Input: part model. Units: mm. Frame: model coordinates. A direction names the side the tool comes from. Give positions to 0.01 mm unless a question says otherwise; leave off trailing zeros. Loops run counter-clockwise (first coordinate to the right, second up) from the corner with the lowest first, then second, coordinate; pieces in that order, holes last.
from build123d import *
from OCP.BRepFilletAPI import BRepFilletAPI_MakeChamfer

# Parameters (mm, degrees)
SKETCH_1_W      = 60
SKETCH_1_H      = 30
EXTRUDE_1_DEPTH = 30
SKETCH_2_W      = 30
SKETCH_2_H      = 30
EXTRUDE_2_DEPTH = 80
EXTRUDE_3_DEPTH = 47
CHAMFER_1_SIZE  = 40
CHAMFER_1_SIZE2 = 7.053079228


with BuildPart() as part:
    # ｽｹｯﾁ1 → ﾎﾞｽ - 押し出し1 (new body)
    with BuildSketch(Plane(origin=(0, 0, 0), x_dir=(1, 0, 0), z_dir=(0, 1, 0))):
        with Locations((30, -15)):
            Rectangle(SKETCH_1_W, SKETCH_1_H)
    extrude(amount=EXTRUDE_1_DEPTH)

    # ｽｹｯﾁ2 → ﾎﾞｽ - 押し出し2 (add)
    with BuildSketch(Plane(origin=(0, 30, 0), x_dir=(1, 0, 0), z_dir=(0, 1, 0))):
        with Locations((15, -15)):
            Rectangle(SKETCH_2_W, SKETCH_2_H)
    extrude(amount=EXTRUDE_2_DEPTH)

    # ｽｹｯﾁ3 → ﾎﾞｽ - 押し出し3 (add)
    with BuildSketch(Plane(origin=(0, 110, 0), x_dir=(1, 0, 0), z_dir=(0, 1, 0))):
        Polygon((4.393398282, -15), (15, -4.393398282), (25.606601718, -15), (15, -25.606601718), align=None)
    extrude(amount=EXTRUDE_3_DEPTH)

    # 面取り1: one chamfer whose edges measure the first distance from different faces: ONE call of the kernel's chamfer builder (chamfer() names one face for all edges)
    chamfer_1_edges_1 = [part.edges().sort_by_distance(p)[0] for p in [
        (9.696699141, 157, 20.303300859),
    ]]
    chamfer_1_side_1 = [part.faces().sort_by_distance(p)[0] for p in [
        (9.696699141, 133.5, 20.303300859),
    ]]
    chamfer_1_edges_2 = [part.edges().sort_by_distance(p)[0] for p in [
        (20.303300859, 157, 20.303300859),
    ]]
    chamfer_1_side_2 = [part.faces().sort_by_distance(p)[0] for p in [
        (20.303300859, 133.5, 20.303300859),
    ]]
    chamfer_1_edges_3 = [part.edges().sort_by_distance(p)[0] for p in [
        (20.303300859, 157, 9.696699141),
    ]]
    chamfer_1_side_3 = [part.faces().sort_by_distance(p)[0] for p in [
        (20.303300859, 133.5, 9.696699141),
    ]]
    chamfer_1_edges_4 = [part.edges().sort_by_distance(p)[0] for p in [
        (9.696699141, 157, 9.696699141),
    ]]
    chamfer_1_side_4 = [part.faces().sort_by_distance(p)[0] for p in [
        (9.696699141, 133.5, 9.696699141),
    ]]
    chamfer_1 = BRepFilletAPI_MakeChamfer(part.part.solid().wrapped)
    for e in chamfer_1_edges_1:
        chamfer_1.Add(CHAMFER_1_SIZE, CHAMFER_1_SIZE2, e.wrapped, chamfer_1_side_1[0].wrapped)  # the first distance lies on this face
    for e in chamfer_1_edges_2:
        chamfer_1.Add(CHAMFER_1_SIZE, CHAMFER_1_SIZE2, e.wrapped, chamfer_1_side_2[0].wrapped)  # the first distance lies on this face
    for e in chamfer_1_edges_3:
        chamfer_1.Add(CHAMFER_1_SIZE, CHAMFER_1_SIZE2, e.wrapped, chamfer_1_side_3[0].wrapped)  # the first distance lies on this face
    for e in chamfer_1_edges_4:
        chamfer_1.Add(CHAMFER_1_SIZE, CHAMFER_1_SIZE2, e.wrapped, chamfer_1_side_4[0].wrapped)  # the first distance lies on this face
    add(Compound.cast(chamfer_1.Shape()), mode=Mode.REPLACE)


solid = part.part
(1) Reachability of faces 1 (the flat face through (20.378, 113.451, 20.229)), 2 (the flat face through (8, 110, 21)), 3 (the flat face through (9.771, 113.451, 20.378)), 4 (the flat face through (45, 30, 15)) from +Z, -Z, +X, -X, +Y, -Y: full face, straight path, thin tool, end or side. Return the list, or none.
Values follow:
face 1: +Z, +X, +Y
face 2: +Y
face 3: +Z, -X, +Y
face 4: +Z, -Z, +X, +Y
(2) Ray query, probe 1 along X at (y, z) = (71, 28.25); probe 2 along Y at (x, z) = (22, 1.5). Return the intervals inside material, ascending.
Values follow:
probe 1: x = 0 to 30
probe 2: y = 0 to 110
(3) Cut plane A-A (z = 7.75). Return the cut outline in (x, y).
Values follow:
outline: (0, 0) - (60, 0) - (60, 30) - (30, 30) - (30, 110) - (18.36, 110) - (18.36, 117) - (15, 130.46) - (11.64, 117) - (11.64, 110) - (0, 110) - close
(4) Pin query (flat end, axial travel): pin 1 Ø10 at (x, y) = (24.5, 102.5) entering from -Z; pin 2 Ø15 at (y, z) = (52, 8) entering from +X. Return the tip coordinate at first contact, or that it passes through.
Values follow:
pin 1: stops at z = 0
pin 2: stops at x = 30
(5) Cut plane B-B (x = 13). Return the cut outline in (y, z), and give its area (3 significant figures).
Values follow:
outline: (0, 0) - (110, 0) - (110, 6.39) - (117, 6.39) - (151.51, 15) - (117, 23.61) - (110, 23.61) - (110, 30) - (0, 30) - close
area: 3,720 mm2
(6) Cut plane C-C (y = 99.5). Return the cut outline in (x, z).
Values follow:
outline: (0, 0) - (30, 0) - (30, 30) - (0, 30) - close
